Input: part model. Units: mm. Frame: model coordinates. A direction names the side the tool comes from. Coordinates: 2 decimals unless noted, no trailing zeros. Loops run counter-clockwise (first coordinate to the right, second up) from the corner with the lowest first, then second, coordinate; pieces in that order, holes last. Notation, with made-up numbers: (-17, 58) - (32, 58) arc R32 cw to (32, 85) - close; hole circle Ø1 at (65.25, 20.5). An arc over 180 degrees is marked (long way). Use one line per item in the form item = value.
from build123d import *

# Parameters (mm, degrees)
BOSS_EXTRUDE1_DEPTH = 300
BOSS_EXTRUDE4_DEPTH = 10
BOSS_EXTRUDE5_DEPTH = 10
FILLET1_R           = 10


with BuildPart() as part:
    # Sketch1 → Boss-Extrude1 (new body)
    with BuildSketch(Plane(origin=(0, 0, 0), x_dir=(0, 0, -1), z_dir=(1, 0, 0))):
        Polygon((0, 0), (0, 100), (150, 100), (150, 200), (300, 200), (300, 300), (450, 300), (450, 400), (600, 400), (600, 500), (750, 500), (750, 0), align=None)
    extrude(amount=BOSS_EXTRUDE1_DEPTH)

    # Sketch5 → Boss-Extrude4 (add)
    with BuildSketch(Plane.ZY):
        Polygon((-750, 500), (-750, 650), (0, 200), (0, 100), (-20, 100), (-20, 188.676192421), (-730, 614.676192421), (-730, 500), align=None)
    extrude(amount=-BOSS_EXTRUDE4_DEPTH)

    # Sketch8 → Boss-Extrude5 (add)
    with BuildSketch(Plane.ZY):
        Polygon((-600, 500), (-600, 536.676192421), (-610, 542.676192421), (-610, 536.676192421), (-610, 500), align=None)
        Polygon((-450, 400), (-450, 446.676192421), (-460, 452.676192421), (-460, 446.676192421), (-460, 400), align=None)
        Polygon((-300, 300), (-300, 356.676192421), (-310, 362.676192421), (-310, 356.676192421), (-310, 300), align=None)
        Polygon((-150, 200), (-150, 266.676192421), (-160, 272.676192421), (-160, 266.676192421), (-160, 200), align=None)
    extrude(amount=-BOSS_EXTRUDE5_DEPTH)

    # Fillet1
    fillet1_edges = [part.edges().sort_by_distance(p)[0] for p in [
        (10, 425, -375),
    ]]
    fillet(fillet1_edges, radius=FILLET1_R - 0.0001)  # a hair under: the kernel refuses the full size


solid = part.part
Q1. Set-up query: faces 5 (the flat face through (4.93, 494.09, -529.02)), 6 (the flat face through (148, 248, -750)). Return all of +Z, -Z, +X, -X, +Y, -Y with unobstructed straight access to the full face (end or side cutting, diameter ignored); none if empty.
Check values:
face_5 = +X, -X
face_6 = -Z, +X, -X, +Y, -Y
Q2. Cut plane B-B, the plane x = 118.5. Return loops of the section in (y, z), then the cut area to 3 significant figures.
Check values:
outline = (0, -750) - (500, -750) - (500, -600) - (400, -600) - (400, -450) - (300, -450) - (300, -300) - (200, -300) - (200, -150) - (100, -150) - (100, 0) - (0, 0) - close
area = 225,000 mm²
Q3. Ray query, line 1 along Y through (x, z) = (171, -626); line 2 along Z through (x, y) = (205.5, 261); line 3 along Y through (x, z) = (243.5, -141). Return the intervals inside material, ascending. Write a range as [from, to].
Check values:
line_1 = [0, 500]
line_2 = [-750, -300]
line_3 = [0, 100]
Q4. Pull-direction query (Y, two-part tool) for faces 1 (the cylindrical face through (7.148, 417.706, -368.689)), 2 (the flat face through (148, 57, 0)), 3 (the flat face through (4.93, 578.17, -669.16)), 4 (the flat face through (4.93, 227.13, -84.09)); classes: pulls with the +Y half, pulls with the -Y half, needs draft (parallel to the pull), parting line crosses it, or undercut.
Check values:
face_1 = pulls with the +Y half
face_2 = needs draft
face_3 = undercut
face_4 = undercut
Q5. Cut plane A-A, the plane y = 148. Return loops of the section in (x, z), then the cut area to 3 significant figures.
Check values:
outline = (0, -750) - (300, -750) - (300, -150) - (0, -150) - close; (0, -20) - (10, -20) - (10, 0) - (0, 0) - close
area = 180,000 mm²
Q6. First-contact query: P1, Ø4, axis at x = 35, y = 492, coming from the +Z side; P2, Ø3, axis at y = 276, z = -549.5, coming from the -X side; P3, Ø12, axis at x = 72.5, y = 298.5, coming from the +Z side; P4, Ø5, axis at x = 6, y = 584, coming from the +Z side. Flat tips, straight axial feed; report the tip coordinate or a pass-through.
Check values:
P1 = -600
P2 = 0
P3 = -300
P4 = -638.72
Q7. Cut plane C-C, the plane y = 415. Give the number of separate pieces and of enclosed holes in the cut face, then the cut area to 3 significant figures.
Check values:
separate_pieces = 3
enclosed_holes = 0
area = 45,400 mm²
